from build123d import *

# Parameters (mm, degrees)
SPROKET_DEPTH       = 9
SKETCH3_R           = 12.5
CUT_EXTRUDE1_DEPTH  = 7
SKETCH4_R           = 10
SKETCH4_R_2         = 7
BOSS_EXTRUDE1_DEPTH = 7
SKETCH5_R           = 8
CUT_EXTRUDE2_DEPTH  = 5.5


with BuildPart() as part:
    # Sprocket → Sproket (new body)
    with BuildSketch(Plane(origin=(-521.333895642, -864.335014518, -1401.843992528), x_dir=(1, 0, 0), z_dir=(0, 0, 1))):
        with BuildLine():
            ThreePointArc((502.621153074, 859.818847383), (503.02864119, 858.378492088), (503.546815178, 856.974153932))
            ThreePointArc((503.546815178, 856.974153932), (503.819037022, 856.702761655), (504.203425444, 856.704771932))
            ThreePointArc((504.203425444, 856.704771932), (509.005673001, 855.369858884), (508.795597259, 850.389955006))
            ThreePointArc((508.795597259, 850.389955006), (508.675219652, 850.024896474), (508.849505331, 849.682284445))
            ThreePointArc((508.849505331, 849.682284445), (510.025789743, 848.756528039), (511.270450563, 847.924969632))
            ThreePointArc((511.270450563, 847.924969632), (511.650203039, 847.865416653), (511.959998194, 848.092980848))
            ThreePointArc((511.959998194, 848.092980848), (516.629740281, 849.835703798), (519.386899492, 845.683397507))
            ThreePointArc((519.386899492, 845.683397507), (519.504087984, 845.317302769), (519.846470359, 845.142566367))
            ThreePointArc((519.846470359, 845.142566367), (521.342250401, 845.085016331), (522.837979924, 845.143864722))
            ThreePointArc((522.837979924, 845.143864722), (523.180210493, 845.318898255), (523.297081161, 845.685094579))
            ThreePointArc((523.297081161, 845.685094579), (526.05063502, 849.839792593), (530.721888079, 848.101123761))
            ThreePointArc((530.721888079, 848.101123761), (531.031880649, 847.873828563), (531.411581288, 847.933711155))
            ThreePointArc((531.411581288, 847.933711155), (532.655519825, 848.766349647), (533.831000211, 849.693126751))
            ThreePointArc((533.831000211, 849.693126751), (534.004988429, 850.035889936), (533.884293987, 850.400843839))
            ThreePointArc((533.884293987, 850.400843839), (533.669895633, 855.380563489), (538.470982641, 856.719644514))
            ThreePointArc((538.470982641, 856.719644514), (538.855372663, 856.717967897), (539.127358829, 856.989596368))
            ThreePointArc((539.127358829, 856.989596368), (539.644313618, 858.394383784), (540.050551314, 859.835092247))
            ThreePointArc((540.050551314, 859.835092247), (539.989839594, 860.214661197), (539.677681217, 860.438972694))
            ThreePointArc((539.677681217, 860.438972694), (536.577223534, 864.341630328), (539.674292437, 868.246977772))
            ThreePointArc((539.674292437, 868.246977772), (539.986255988, 868.471560146), (540.046638209, 868.851181652))
            ThreePointArc((540.046638209, 868.851181652), (539.639150093, 870.291536947), (539.120976106, 871.695875104))
            ThreePointArc((539.120976106, 871.695875104), (538.848754261, 871.967267381), (538.464365839, 871.965257104))
            ThreePointArc((538.464365839, 871.965257104), (533.662118282, 873.300170152), (533.872194024, 878.280074029))
            ThreePointArc((533.872194024, 878.280074029), (533.992571631, 878.645132562), (533.818285952, 878.98774459))
            ThreePointArc((533.818285952, 878.98774459), (532.642001541, 879.913500997), (531.39734072, 880.745059403))
            ThreePointArc((531.39734072, 880.745059403), (531.017588244, 880.804612382), (530.70779309, 880.577048188))
            ThreePointArc((530.70779309, 880.577048188), (526.038051002, 878.834325238), (523.280891791, 882.986631528))
            ThreePointArc((523.280891791, 882.986631528), (523.163703299, 883.352726267), (522.821320924, 883.527462669))
            ThreePointArc((522.821320924, 883.527462669), (521.325540883, 883.585012705), (519.829811359, 883.526164313))
            ThreePointArc((519.829811359, 883.526164313), (519.48758079, 883.35113078), (519.370710122, 882.984934457))
            ThreePointArc((519.370710122, 882.984934457), (516.617156263, 878.830236442), (511.945903204, 880.568905275))
            ThreePointArc((511.945903204, 880.568905275), (511.635910634, 880.796200472), (511.256209995, 880.736317881))
            ThreePointArc((511.256209995, 880.736317881), (510.012271459, 879.903679389), (508.836791072, 878.976902284))
            ThreePointArc((508.836791072, 878.976902284), (508.662802855, 878.6341391), (508.783497297, 878.269185196))
            ThreePointArc((508.783497297, 878.269185196), (508.99789565, 873.289465546), (504.196808642, 871.950384521))
            ThreePointArc((504.196808642, 871.950384521), (503.81241862, 871.952061138), (503.540432454, 871.680432668))
            ThreePointArc((503.540432454, 871.680432668), (503.023477665, 870.275645251), (502.617239969, 868.834936788))
            ThreePointArc((502.617239969, 868.834936788), (502.677951689, 868.455367839), (502.990110067, 868.231056341))
            ThreePointArc((502.990110067, 868.231056341), (506.090567749, 864.328398708), (502.993498846, 860.423051264))
            ThreePointArc((502.993498846, 860.423051264), (502.681535295, 860.198468889), (502.621153074, 859.818847383))
        make_face()
    sproket = extrude(amount=SPROKET_DEPTH)

    # Sketch3 → Cut-Extrude1 (cut)
    with BuildSketch(Plane.XY.offset(-1392.843992528)):
        Circle(SKETCH3_R)
    cut_extrude1 = extrude(amount=-CUT_EXTRUDE1_DEPTH, mode=Mode.SUBTRACT)

    # Mirror1: Sproket, Cut-Extrude1 across plane
    add(sproket.mirror(Plane(origin=(9.113348653, 2.199432046, -1401.843992528), x_dir=(1, 0, 0), z_dir=(0, 0, 1))))
    add(cut_extrude1.mirror(Plane(origin=(9.113348653, 2.199432046, -1401.843992528), x_dir=(1, 0, 0), z_dir=(0, 0, 1))), mode=Mode.SUBTRACT)

    # Sketch4 → Boss-Extrude1 (add)
    with BuildSketch(Plane(origin=(0, 0, -1403.843992528), x_dir=(-1, 0, 0), z_dir=(0, 0, -1))):
        Circle(SKETCH4_R)
        Circle(SKETCH4_R_2, mode=Mode.SUBTRACT)
    extrude(amount=BOSS_EXTRUDE1_DEPTH)

    # Sketch5 → Cut-Extrude2 (cut)
    with BuildSketch(Plane.XY.offset(-1399.843992528)):
        Circle(SKETCH5_R)
    extrude(amount=-CUT_EXTRUDE2_DEPTH, mode=Mode.SUBTRACT)


solid = part.part
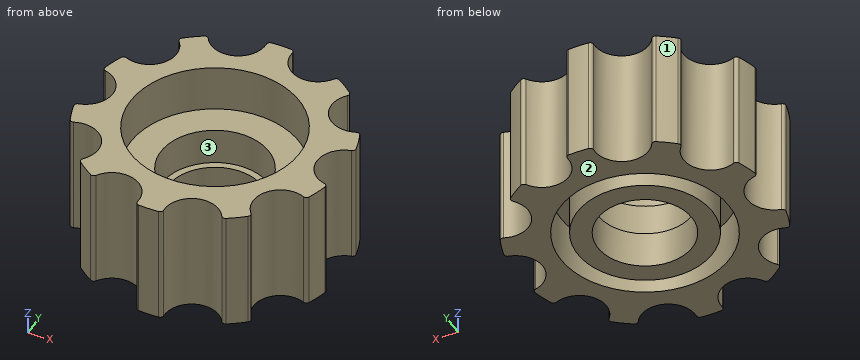
Verification items for the finished model (mm, model axes). Face numbers are marked on the shaded views. Coordinates: 2 decimals unless noted, no trailing zeros. Order: outer loops, then holes, each group sorted by start corner. A loop starts at its lowest first (then second) coordinate and runs counter-clockwise, first axis right, second up.
1. Go/stop test with flat-tipped pins: pin 1 Ø1 at (x, z) = (13.5, -1408) entering from -Y; pin 2 Ø21 at (x, y) = (0, 0) entering from +Z; pin 3 Ø6 at (y, z) = (15.5, -1405.5) entering from +X. Record where each tip stops, or that it passes through.
Results found:
pin 1: stops at y = -8.24
pin 2: stops at z = -1399.84
pin 3: stops at x = 12.66
2. Sectioned sample at C-C, the plane z = -1409.5. Give the number of separate pieces and of enclosed holes in the cut face, and give its area (3 significant figures).
Results found:
separate pieces: 2
enclosed holes: 2
area: 591 mm2
3. Sectioned sample at A-A, the plane y = 0. Record the cut outline in (x, z).
Results found:
outline: (-15.24, -1410.84) - (-12.5, -1410.84) - (-12.5, -1403.84) - (-10, -1403.84) - (-10, -1410.84) - (-7, -1410.84) - (-7, -1405.34) - (-8, -1405.34) - (-8, -1399.84) - (-12.5, -1399.84) - (-12.5, -1392.84) - (-15.24, -1392.84) - close; (7, -1410.84) - (10, -1410.84) - (10, -1403.84) - (12.5, -1403.84) - (12.5, -1410.84) - (15.24, -1410.84) - (15.24, -1392.84) - (12.5, -1392.84) - (12.5, -1399.84) - (8, -1399.84) - (8, -1405.34) - (7, -1405.34) - close
4. Scan lines: line 1 (Y direction, x = 0, z = -1402.8); line 2 (Y direction, x = 0, z = -1394.5); line 3 (X direction, y = 3, z = -1407.25). Record each from-to range of solid material in increasing order.
Results found:
line 1: y = -19.25 to -8, 8 to 19.25
line 2: y = -19.25 to -12.5, 12.5 to 19.25
line 3: x = -16.6 to -12.13, -9.54 to -6.32, 6.32 to 9.54, 12.13 to 16.58
5. Release check for a two-part mould opening along Y. For the marked faces 1, 2 and 3 record: +Y half, -Y half, draft (parallel to the pull), parting line (faces both ways), or undercut.
Results found:
face 1: +Y half
face 2: draft
face 3: undercut
6. Sectioned sample at B-B, the plane x = 0. Record the cut outline in (y, z).
Results found:
outline: (-19.25, -1410.84) - (-12.5, -1410.84) - (-12.5, -1403.84) - (-10, -1403.84) - (-10, -1410.84) - (-7, -1410.84) - (-7, -1405.34) - (-8, -1405.34) - (-8, -1399.84) - (-12.5, -1399.84) - (-12.5, -1392.84) - (-19.25, -1392.84) - close; (7, -1410.84) - (10, -1410.84) - (10, -1403.84) - (12.5, -1403.84) - (12.5, -1410.84) - (19.25, -1410.84) - (19.25, -1392.84) - (12.5, -1392.84) - (12.5, -1399.84) - (8, -1399.84) - (8, -1405.34) - (7, -1405.34) - close
7. Sectioned sample at D-D, the plane y = -10.5. Record the cut outline in (x, z).
Results found:
outline: (-11.65, -1410.84) - (-6.78, -1410.84) - (-6.78, -1403.84) - (6.78, -1403.84) - (6.78, -1410.84) - (11.65, -1410.84) - (11.65, -1392.84) - (6.78, -1392.84) - (6.78, -1399.84) - (-6.78, -1399.84) - (-6.78, -1392.84) - (-11.65, -1392.84) - close
